Could you check a few things on this model? Use its own coordinates, in mm. A direction names the side the tool comes from. Give positions to 0.01 mm unless a question says otherwise; leave off trailing zeros. Order: outer loops, then holes, each group sorted by start corner. A loop starts at its lowest first (then second) coordinate and runs counter-clockwise, first axis right, second up. Notation, with made-up numbers: M 60.5,61.5 L 95.5,61.5 A15 cw 95.5,85.5 Z; hole C -39.5,6 d9. An arc over 180 degrees is marked long. Use a Markdown table: item, result. Add a question column.
Item 1: Suppose I cut it at B-B on x = 0.6. Count the separate pieces of the cut face and the enclosed holes in it, plus the area to 3 significant figures.
Item 2: If we mould it in two halves opening along Y, with no side actions, what happens to faces 6 (the face through (2, -3, -26)), 7 (the face through (2, 25, -140)), 8 (the face through (2, 34, -6)), 9 (the face through (2, 32.9, -40))? For each: released by +Y, released by -Y, zero draft, split by the parting line, or undercut.
Item 3: Suppose I cut it at A-A on z = -117.5. Write out the boundary of the cut face in (x, y), plus the area to 3 significant figures.
Item 4: If I drill on L1, parallel to Y at x = 0.8, z = -41; L2, parallel to Z at x = 0.8, y = 71.5; L3, parallel to Y at x = 0.4, z = -102, over which ranges is the centre line in solid material (lowest first)? Write a range as from..to.
Item 5: Suppose I cut it at C-C on y = 15. Write out the boundary of the cut face in (x, z).
Item 6: I'm going to push flat-ended pins straight in: pin 1 Ø1.5 at (x, z) = (1.5, -83) entering from -Y; pin 2 Ø1.5 at (x, y) = (2, -1) entering from +Z. Where does each tip first touch, or does it pass through?
Item 7: For faces 1 (the face through (1, 38, 0)), 2 (the face through (2, 50, -139)), 3 (the face through (2, 29.8, -103)), 4 (the face through (2, 65, -140)), 5 (the face through (2, -1, -87.5)), which set-ups out of +Z, -Z, +X, -X, +Y, -Y let a thin tool reach every point of the face, with its end or its side?
Autodesk Inventor part; units mm, degrees
ref_plane "YZ Plane" through (0, 0, 0) normal (1, 0, 0) x (0, 1, 0)
ref_plane "XZ Plane" through (0, 0, 0) normal (0, 1, 0) x (-1, 0, 0)
ref_plane "XY Plane" through (0, 0, 0) normal (0, 0, 1) x (1, 0, 0)
sketch "Sketch1" plane through (0, 0, 0) normal (1, 0, 0) x (0, 1, 0)
  line L0 (0, 0) -> (77, 0)
  line L1 (77, 0) -> (77, -140)
  line L2 (77, -140) -> (0, -140)
  line L3 (0, 0) -> (-3, 0)
  line L4 (-3, 0) -> (-3, -140)
  line L5 (-3, -140) -> (0, -140)
  dimension "d1" = 140
extrude "Extrusion1" add sketch "Sketch1" along normal blind 3
sketch "Sketch5" plane through (3, 0, 0) normal (1, 0, 0) x (0, 0, -1)
  line L0 (6, 73.9) -> (6, 70.9)
  line L1 (6, 70.9) -> (10, 70.9)
  line L2 (10, 70.9) -> (10, 73.9)
  line L3 (10, 73.9) -> (6, 73.9)
  line L4 (0, 77) -> (0, 0)
  line L5 (140, 77) -> (0, 77)
  line L6 (37.75, 73.9) -> (37.75, 70.9)
  line L7 (37.75, 70.9) -> (41.75, 70.9)
  line L8 (41.75, 70.9) -> (41.75, 73.9)
  line L9 (41.75, 73.9) -> (37.75, 73.9)
  line L10 (6, 35.9) -> (6, 32.9)
  line L11 (6, 32.9) -> (10, 32.9)
  line L12 (10, 32.9) -> (10, 35.9)
  line L13 (10, 35.9) -> (6, 35.9)
  line L14 (37.75, 35.9) -> (37.75, 32.9)
  line L15 (37.75, 32.9) -> (41.75, 32.9)
  line L16 (41.75, 32.9) -> (41.75, 35.9)
  line L17 (41.75, 35.9) -> (37.75, 35.9)
  line L18 (69.5, 73.9) -> (69.5, 70.9)
  line L19 (69.5, 70.9) -> (73.5, 70.9)
  line L20 (73.5, 70.9) -> (73.5, 73.9)
  line L21 (73.5, 73.9) -> (69.5, 73.9)
  line L22 (69.5, 35.9) -> (69.5, 32.9)
  line L23 (69.5, 32.9) -> (73.5, 32.9)
  line L24 (73.5, 32.9) -> (73.5, 35.9)
  line L25 (73.5, 35.9) -> (69.5, 35.9)
  line L26 (101.25, 73.9) -> (101.25, 70.9)
  line L27 (101.25, 70.9) -> (105.25, 70.9)
  line L28 (105.25, 70.9) -> (105.25, 73.9)
  line L29 (105.25, 73.9) -> (101.25, 73.9)
  line L30 (101.25, 35.9) -> (101.25, 32.9)
  line L31 (101.25, 32.9) -> (105.25, 32.9)
  line L32 (105.25, 32.9) -> (105.25, 35.9)
  line L33 (105.25, 35.9) -> (101.25, 35.9)
  line L34 (133, 73.9) -> (133, 70.9)
  line L35 (133, 70.9) -> (137, 70.9)
  line L36 (137, 70.9) -> (137, 73.9)
  line L37 (137, 73.9) -> (133, 73.9)
  line L38 (133, 35.9) -> (133, 32.9)
  line L39 (133, 32.9) -> (137, 32.9)
  line L40 (137, 32.9) -> (137, 35.9)
  line L41 (137, 35.9) -> (133, 35.9)
  line L42 (10, 26.8) -> (10, 29.8)
  line L43 (10, 29.8) -> (6, 29.8)
  line L44 (6, 26.8) -> (10, 26.8)
  line L45 (6, 29.8) -> (6, 26.8)
  line L46 (69.5, 29.8) -> (69.5, 26.8)
  line L47 (69.5, 26.8) -> (73.5, 26.8)
  line L48 (73.5, 29.8) -> (69.5, 29.8)
  line L49 (73.5, 26.8) -> (73.5, 29.8)
  line L50 (41.75, 29.8) -> (37.75, 29.8)
  line L51 (37.75, 26.8) -> (41.75, 26.8)
  line L52 (41.75, 26.8) -> (41.75, 29.8)
  line L53 (37.75, 29.8) -> (37.75, 26.8)
  line L54 (133, 29.8) -> (133, 26.8)
  line L55 (137, 29.8) -> (133, 29.8)
  line L56 (133, 26.8) -> (137, 26.8)
  line L57 (137, 26.8) -> (137, 29.8)
  line L58 (101.25, 29.8) -> (101.25, 26.8)
  line L59 (101.25, 26.8) -> (105.25, 26.8)
  line L60 (105.25, 26.8) -> (105.25, 29.8)
  line L61 (105.25, 29.8) -> (101.25, 29.8)
  line L62 (140, -3) -> (140, 77)
  dimension "d67" = 3
  dimension "d68" = 4
  dimension "d93" = 3.1
  dimension "d97" = 6
  dimension "d100" = 31.75
  dimension "d103" = 38
  dimension "d108" = 6.1
  dimension "d113" = 3
extrude "Extrusion5" cut sketch "Sketch5" against normal blind 10
sketch "Sketch6" plane through (3, 0, 0) normal (1, 0, 0) x (0, 0, -1)
  line L0 (0, 0) -> (17.5, 0)
  line L1 (17.5, 0) -> (17.5, -3)
  line L2 (17.5, -3) -> (35, -3)
  line L3 (35, -3) -> (35, 0)
  line L4 (0, 0) -> (0, 10)
  line L5 (140, 0) -> (140, 9.94)
  line L6 (137, 9.94) -> (137, 19.94)
  line L7 (137, 19.94) -> (140, 19.94)
  line L8 (140, 30) -> (137, 30)
  line L9 (137, 30) -> (137, 40)
  line L10 (137, 40) -> (140, 40)
  line L11 (140, 40) -> (140, 50)
  line L12 (140, 50) -> (137, 50)
  line L13 (137, 50) -> (137, 60)
  line L14 (137, 60) -> (140, 60)
  line L15 (140, 60) -> (140, 70)
  line L16 (140, 70) -> (137, 70)
  line L17 (137, 70) -> (137, 77)
  line L18 (140, 9.94) -> (137, 9.94)
  line L19 (140, 19.94) -> (140, 30)
  line L20 (3, 77) -> (137, 77)
  line L21 (0, 77) -> (0, 0)
  line L22 (0, 0) -> (0, 77)
  line L23 (0, 77) -> (3, 77)
  line L24 (35, 0) -> (52.5, 0)
  line L25 (52.5, 0) -> (52.5, -3)
  line L26 (52.5, -3) -> (70, -3)
  line L27 (70, -3) -> (70, 0)
  line L28 (70, 0) -> (87.5, 0)
  line L29 (87.5, 0) -> (87.5, -3)
  line L30 (87.5, -3) -> (105, -3)
  line L31 (105, -3) -> (105, 0)
  line L32 (105, 0) -> (122.5, 0)
  line L33 (122.5, 0) -> (122.5, -3)
  line L34 (122.5, -3) -> (140, -3)
  line L35 (140, 30) -> (140, 19.94)
  line L36 (140, 9.94) -> (140, -3)
  line L37 (140, 40) -> (140, 50)
  line L38 (140, 60) -> (140, 70)
  line L39 (140, -3) -> (140, 9.94)
  line L40 (137, 9.94) -> (137, 19.94)
  line L41 (0, 0) -> (0, 77)
  line L42 (137, 77) -> (0, 77)
  line L43 (0, 77) -> (0, 10)
  point P0 (0, 70)
extrude "Extrusion6" cut sketch "Sketch6" against normal blind 3 keep common part
properties part number "DoosjeRechterkant" material "Wood (Cherry)"
Findings below:
| question | item | result |
|---|---|---|
| 1 | separate pieces | 1 |
| 1 | enclosed holes | 13 |
| 1 | area | 10,700 mm^2 |
| 2 | face 6 | released by -Y |
| 2 | face 7 | zero draft |
| 2 | face 8 | undercut |
| 2 | face 9 | undercut |
| 3 | outline | M 0,0 L 3,0 L 3,77 L 0,77 Z |
| 3 | area | 231 mm^2 |
| 4 | L1 | y = 0..26.8, 29.8..32.9, 35.9..70.9, 73.9..77 |
| 4 | L2 | z = -133..-105.25, -101.25..-73.5, -69.5..-41.75, -37.75..-10, -6..0 |
| 4 | L3 | y = -3..26.8, 29.8..32.9, 35.9..70.9, 73.9..77 |
| 5 | outline | M 0,-137 L 3,-137 L 3,0 L 0,0 Z |
| 6 | pin 1 | stops at y = 0 |
| 6 | pin 2 | stops at z = -17.5 |
| 7 | face 1 | +Z, +X, -X, +Y, -Y |
| 7 | face 2 | -Z, +X, -X |
| 7 | face 3 | +X, -X |
| 7 | face 4 | -Z, +X, -X, +Y, -Y |
| 7 | face 5 | +X, -X, -Y |
